Design review of the part built by this model. Coordinates are the model's own, in mm. Face numbers are marked on the shaded views. A direction names the side the tool comes from. Coordinates: 2 decimals unless noted, no trailing zeros. Loops run counter-clockwise (first coordinate to the right, second up) from the corner with the lowest first, then second, coordinate; pieces in that order, holes last. Notation, with made-up numbers: M 62.25,11 L 104.25,11 A19 ccw 104.25,19 Z; hole C 6.5,34.5 d6. An arc over 180 degrees is marked long. Answer as a JSON object with one key per item and string values. Group by question number.
1. Draft analysis for pull direction X (two halves, no side actions). For the marked faces 3 and 4, state which applies: +X half, -X half, draft (parallel to the pull), parting line (faces both ways), or undercut.
2. Consider section A-A (x = 20). Count the separate pieces of the cut face and the enclosed holes in it, then the cut area to 3 significant figures.
3. To check wall thickness, follow probe 1 along Z at (x, y) = (18, -22); probe 2 along Z at (x, y) = (15, -14); probe 3 along Z at (x, y) = (3.5, -17.5). State the ranges of each line that lie inside material, in increasing order.
4. Consider section B-B (z = 43). State the section outline as (x, y) points, then the cut area to 3 significant figures.
5. Insertion check: pin 1 (1.3 mm diameter, centred on y = -5.5, z = -51, fed in from -X); pin 2 (6 mm diameter, centred on x = 7, z = -53, fed in from +Y); pin 3 (1.3 mm diameter, centred on y = -5.5, z = -52, fed in from +X). Each pin has a flat end and moves straight along its axis. Give the tip position at first contact, or say it passes through.
6. Machinability: for the marked faces 1 and 2, which of the approach directions +Z, -Z, +X, -X, +Y, -Y give a long, thin tool a straight path to every point of the face, cutting with its end or side? Answer none if there is none.
from build123d import *

# Parameters (mm, degrees)
F1_DEPTH  = 60
F2_DEPTH  = 5
F3_DEPTH  = 60
F4_R      = 5
F7_DEPTH  = 5
F8_DEPTH  = 5
F9_DEPTH  = 1
F10_DEPTH = 1
F12_DEPTH = 25
F13_DEPTH = 20
F14_DEPTH = 10


with BuildPart() as f1:
    # F0 (on Right) → F1 (new body)
    with BuildSketch(Plane.YZ):
        Polygon((-1.9545168432, 38.6489601963), (-33.5964987424, 14.1788767986), (-28.2257758369, -25.4589250511), (-8.406874912, -22.7735635983), (-0.7535947717, -79.2574312341), (4.2011304595, -78.5860908709), (-3.9713255886, -18.2705245759), (3.1545996335, -0.8816359607), (10.2805248557, 16.5072526545), (58.4291094867, 53.742590351), (55.370349062, 57.6978380884), (10.2805248557, 22.8279692467), align=None)
        Polygon((-25.8654488138, -5.6400241263), (-7.3142972833, -13.2422419285), (-9.1963342424, -17.8348428934), (-23.9423909688, -19.8328594567), align=None, mode=Mode.SUBTRACT)
        Polygon((1.5615552233, 8.4168698067), (-1.4719884671, 1.0143288458), (-4.5055321574, -6.3882121151), (-5.26391808, -8.2388473554), (-11.7411414209, -5.5844966263), (-17.2930471416, -3.3093388585), (-23.7702704824, -0.6549881294), (-23.0118845598, 1.1956471108), (-16.944797179, 16.0007290327), (-16.1864112564, 17.851364273), (-9.7091879156, 15.1970135439), (-4.1572821949, 12.9218557761), (2.3199411459, 10.267505047), align=None, mode=Mode.SUBTRACT)
        Polygon((-14.6534166938, 22.50764705), (-2.8510041559, 31.6349520341), (6.2523573083, 19.863500585), (4.1741345282, 14.7921613112), align=None, mode=Mode.SUBTRACT)
    extrude(amount=F1_DEPTH)

    # F0 (on Right) → F2 (join)
    with BuildSketch(Plane.YZ):
        Polygon((-16.944797179, 16.0007290327), (-10.4675738382, 13.3463783036), (-9.7091879156, 15.1970135439), (-16.1864112564, 17.851364273), align=None)
        Polygon((-4.9156681175, 11.0712205358), (1.5615552233, 8.4168698067), (2.3199411459, 10.267505047), (-4.1572821949, 12.9218557761), align=None)
        Polygon((-5.26391808, -8.2388473554), (-4.5055321574, -6.3882121151), (-10.9827554983, -3.7338613861), (-11.7411414209, -5.5844966263), align=None)
        Polygon((-17.2930471416, -3.3093388585), (-16.534661219, -1.4587036183), (-23.0118845598, 1.1956471108), (-23.7702704824, -0.6549881294), align=None)
    extrude(amount=F2_DEPTH)

    # F0 (on Right) → F3 (join)
    with BuildSketch(Plane.YZ):
        Polygon((-11.7411414209, -5.5844966263), (-10.9827554983, -3.7338613861), (-16.534661219, -1.4587036183), (-17.2930471416, -3.3093388585), align=None)
        Polygon((-10.4675738382, 13.3463783036), (-4.9156681175, 11.0712205358), (-4.1572821949, 12.9218557761), (-9.7091879156, 15.1970135439), align=None)
    extrude(amount=F3_DEPTH)

    # F4
    f4_edges = [f1.edges().sort_by_distance(p)[0] for p in [
        (30, -33.596499, 14.178877),
    ]]
    fillet(f4_edges, radius=F4_R)

    # F6 (on face) → F7 (cut)
    with BuildSketch(Plane(origin=(0, -11.2853910764, -1.5291137632), x_dir=(1, 0, 0), z_dir=(0, -0.9909450462, -0.1342680726))):
        with BuildLine():
            ThreePointArc((7.9984828914, -64.1860215089), (9.9984828914, -66.1860215089), (11.9984828914, -64.1860215089))
            ThreePointArc((11.9984828914, -64.1860215089), (9.9984828914, -62.1860215089), (7.9984828914, -64.1860215089))
        make_face()
        with BuildLine():
            ThreePointArc((7.9984828914, -35.6860233554), (9.9984828914, -37.6860233554), (11.9984828914, -35.6860233554))
            ThreePointArc((11.9984828914, -35.6860233554), (9.9984828914, -33.6860233554), (7.9984828914, -35.6860233554))
        make_face()
        with BuildLine():
            ThreePointArc((48.0015171086, -35.6972638628), (50.0015171086, -37.6972638628), (52.0015171086, -35.6972638628))
            ThreePointArc((52.0015171086, -35.6972638628), (50.0015171086, -33.6972638628), (48.0015171086, -35.6972638628))
        make_face()
        with BuildLine():
            ThreePointArc((48.0015171086, -64.1849918396), (50.0015171086, -66.1849918396), (52.0015171086, -64.1849918396))
            ThreePointArc((52.0015171086, -64.1849918396), (50.0015171086, -62.1849918396), (48.0015171086, -64.1849918396))
        make_face()
    extrude(amount=-F7_DEPTH, mode=Mode.SUBTRACT)

    # F5 (on face) → F8 (cut)
    with BuildSketch(Plane(origin=(0, -7.1996627103, 9.3098006026), x_dir=(1, 0, 0), z_dir=(0, -0.6117520849, 0.7910495475))):
        with BuildLine():
            ThreePointArc((48, 66.4655810893), (50, 64.4655810893), (52, 66.4655810893))
            ThreePointArc((52, 66.4655810893), (50, 68.4655810893), (48, 66.4655810893))
        make_face()
        with BuildLine():
            ThreePointArc((48, 37.9655810893), (50, 35.9655810893), (52, 37.9655810893))
            ThreePointArc((52, 37.9655810893), (50, 39.9655810893), (48, 37.9655810893))
        make_face()
        with BuildLine():
            ThreePointArc((8, 37.9655810893), (10, 35.9655810893), (12, 37.9655810893))
            ThreePointArc((12, 37.9655810893), (10, 39.9655810893), (8, 37.9655810893))
        make_face()
        with BuildLine():
            ThreePointArc((8, 66.4655810893), (10, 64.4655810893), (12, 66.4655810893))
            ThreePointArc((12, 66.4655810893), (10, 68.4655810893), (8, 66.4655810893))
        make_face()
    extrude(amount=-F8_DEPTH, mode=Mode.SUBTRACT)

    # F5 (on face) → F9 (join)
    with BuildSketch(Plane(origin=(0, -7.1996627103, 9.3098006026), x_dir=(1, 0, 0), z_dir=(0, -0.6117520849, 0.7910495475))):
        with BuildLine():
            ThreePointArc((48, 58.4655810893), (50, 56.4655810893), (52, 58.4655810893))
            ThreePointArc((52, 58.4655810893), (50, 60.4655810893), (48, 58.4655810893))
        make_face()
        with BuildLine():
            Line((52, 45.9655810893), (52, 58.4655810893))
            ThreePointArc((52, 58.4655810893), (50, 56.4655810893), (48, 58.4655810893))
            Line((48, 58.4655810893), (48, 45.9655810893))
            ThreePointArc((48, 45.9655810893), (50, 47.9655810893), (52, 45.9655810893))
        make_face()
        with BuildLine():
            ThreePointArc((48, 45.9655810893), (50, 43.9655810893), (52, 45.9655810893))
            ThreePointArc((52, 45.9655810893), (50, 47.9655810893), (48, 45.9655810893))
        make_face()
        with BuildLine():
            ThreePointArc((8, 58.4655810893), (10, 56.4655810893), (12, 58.4655810893))
            ThreePointArc((12, 58.4655810893), (10, 60.4655810893), (8, 58.4655810893))
        make_face()
        with BuildLine():
            ThreePointArc((8, 45.9655810893), (10, 47.9655810893), (12, 45.9655810893))
            Line((12, 45.9655810893), (12, 58.4655810893))
            ThreePointArc((12, 58.4655810893), (10, 56.4655810893), (8, 58.4655810893))
            Line((8, 58.4655810893), (8, 45.9655810893))
        make_face()
        with BuildLine():
            ThreePointArc((8, 45.9655810893), (10, 43.9655810893), (12, 45.9655810893))
            ThreePointArc((12, 45.9655810893), (10, 47.9655810893), (8, 45.9655810893))
        make_face()
    extrude(amount=F9_DEPTH)

    # F6 (on face) → F10 (join)
    with BuildSketch(Plane(origin=(0, -11.2853910764, -1.5291137632), x_dir=(1, 0, 0), z_dir=(0, -0.9909450462, -0.1342680726))):
        with BuildLine():
            ThreePointArc((48.0015171086, -43.6972638628), (50.0015171086, -45.6972638628), (52.0015171086, -43.6972638628))
            ThreePointArc((52.0015171086, -43.6972638628), (50.0015171086, -41.6972638628), (48.0015171086, -43.6972638628))
        make_face()
        with BuildLine():
            Line((52.0015171086, -56.1849918396), (52.0015171086, -43.6972638628))
            ThreePointArc((52.0015171086, -43.6972638628), (50.0015171086, -45.6972638628), (48.0015171086, -43.6972638628))
            Line((48.0015171086, -43.6972638628), (48.0015171086, -56.1849918396))
            ThreePointArc((48.0015171086, -56.1849918396), (50.0015171086, -54.1849918396), (52.0015171086, -56.1849918396))
        make_face()
        with BuildLine():
            ThreePointArc((48.0015171086, -56.1849918396), (50.0015171086, -58.1849918396), (52.0015171086, -56.1849918396))
            ThreePointArc((52.0015171086, -56.1849918396), (50.0015171086, -54.1849918396), (48.0015171086, -56.1849918396))
        make_face()
        with BuildLine():
            ThreePointArc((7.9984828914, -43.6860233554), (9.9984828914, -45.6860233554), (11.9984828914, -43.6860233554))
            ThreePointArc((11.9984828914, -43.6860233554), (9.9984828914, -41.6860233554), (7.9984828914, -43.6860233554))
        make_face()
        with BuildLine():
            ThreePointArc((7.9984828914, -56.1860215089), (9.9984828914, -54.1860215089), (11.9984828914, -56.1860215089))
            Line((11.9984828914, -56.1860215089), (11.9984828914, -43.6860233554))
            ThreePointArc((11.9984828914, -43.6860233554), (9.9984828914, -45.6860233554), (7.9984828914, -43.6860233554))
            Line((7.9984828914, -43.6860233554), (7.9984828914, -56.1860215089))
        make_face()
        with BuildLine():
            ThreePointArc((7.9984828914, -56.1860215089), (9.9984828914, -58.1860215089), (11.9984828914, -56.1860215089))
            ThreePointArc((11.9984828914, -56.1860215089), (9.9984828914, -54.1860215089), (7.9984828914, -56.1860215089))
        make_face()
    extrude(amount=F10_DEPTH)

    # F11 (on face) → F12 (cut)
    with BuildSketch(Plane(origin=(0, -20.1225891662, 8.2461892101), x_dir=(-1, 0, 0), z_dir=(0, 0.9253176201, -0.3791929613))):
        with BuildLine():
            Line((-12, 0.3804086878), (-8, 0.3804086878))
            ThreePointArc((-8, 0.3804086878), (-10, 2.3804086878), (-12, 0.3804086878))
        make_face()
        with BuildLine():
            Line((-52, 0.3804086878), (-48, 0.3804086878))
            ThreePointArc((-48, 0.3804086878), (-50, 2.3804086878), (-52, 0.3804086878))
        make_face()
        with BuildLine():
            ThreePointArc((-52, 0.3804086878), (-50, -1.6195913122), (-48, 0.3804086878))
            Line((-48, 0.3804086878), (-52, 0.3804086878))
        make_face()
        with BuildLine():
            ThreePointArc((-12, 0.3804086878), (-10, -1.6195913122), (-8, 0.3804086878))
            Line((-8, 0.3804086878), (-12, 0.3804086878))
        make_face()
    extrude(amount=-F12_DEPTH, mode=Mode.SUBTRACT)

    # F11 (on face) → F13 (join)
    with BuildSketch(Plane(origin=(0, -20.1225891662, 8.2461892101), x_dir=(-1, 0, 0), z_dir=(0, 0.9253176201, -0.3791929613))):
        with BuildLine():
            Line((-48, 0.3804086878), (-46, 0.3804086878))
            ThreePointArc((-46, 0.3804086878), (-50, 4.3804086878), (-54, 0.3804086878))
            Line((-54, 0.3804086878), (-52, 0.3804086878))
            ThreePointArc((-52, 0.3804086878), (-50, 2.3804086878), (-48, 0.3804086878))
        make_face()
        with BuildLine():
            ThreePointArc((-54, 0.3804086878), (-50, -3.6195913122), (-46, 0.3804086878))
            Line((-46, 0.3804086878), (-48, 0.3804086878))
            ThreePointArc((-48, 0.3804086878), (-50, -1.6195913122), (-52, 0.3804086878))
            Line((-52, 0.3804086878), (-54, 0.3804086878))
        make_face()
        with BuildLine():
            ThreePointArc((-14, 0.3804086878), (-10, -3.6195913122), (-6, 0.3804086878))
            Line((-6, 0.3804086878), (-8, 0.3804086878))
            ThreePointArc((-8, 0.3804086878), (-10, -1.6195913122), (-12, 0.3804086878))
            Line((-12, 0.3804086878), (-14, 0.3804086878))
        make_face()
        with BuildLine():
            Line((-8, 0.3804086878), (-6, 0.3804086878))
            ThreePointArc((-6, 0.3804086878), (-10, 4.3804086878), (-14, 0.3804086878))
            Line((-14, 0.3804086878), (-12, 0.3804086878))
            ThreePointArc((-12, 0.3804086878), (-10, 2.3804086878), (-8, 0.3804086878))
        make_face()
    extrude(amount=-F13_DEPTH)

    # F14 (cut): faces of the model
    f14_faces = [f1.faces().sort_by_distance(p)[0] for p in [
        (7.886862915, -38.4846932718, 16.1820472977),
        (46.113137085, -38.4846932718, 16.1820472977),
    ]]
    extrude(f14_faces, amount=-F14_DEPTH, mode=Mode.SUBTRACT)


solid = f1.part
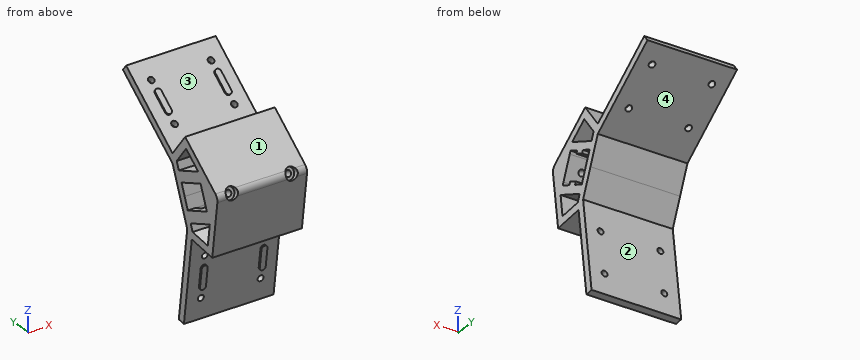
Findings below:
{
 "1": {"face 3": "undercut", "face 4": "draft"},
 "2": {"separate pieces": "1", "enclosed holes": "3", "area": "1,710 mm^2"},
 "3": {"probe 1": "z = -24.62 to -19.57, -7.22 to -1.38, 3.66 to 23.15", "probe 2": "z = -23.53 to -18.49, -10.5 to -2.5, 16.96 to 22.24, 23.01 to 29.33", "probe 3": "z = -24.01 to -18.96, -9.07 to -1.06, 14.65 to 26.63"},
 "4": {"outline": "M 0,36.36 L 8,36.36 L 8,34.73 L 12,34.73 L 12,36.36 L 48,36.36 L 48,34.73 L 52,34.73 L 52,36.36 L 60,36.36 L 60,44.54 L 0,44.54 Z", "area": "503 mm^2"},
 "5": {"pin 1": "stops at x = 8", "pin 2": "stops at y = 1.14", "pin 3": "stops at x = 52"},
 "6": {"face 1": "+Z, +X, -X, -Y", "face 2": "+X, -X, +Y"}
}
